Drawing for the job (mm, zero at the part's lowest x, y, z). Give positions to 0.01 mm unless a question says otherwise; leave off trailing zeros. Write each loop counter-clockwise with the first axis right and the second up, starting at its lowest first coordinate (ties: lowest second). Pieces come first, ordered by that corner, then holes. Notation, with made-up numbers: (46.5, 37.5) - (70.5, 37.5) arc R16 cw to (70.5, 59.5) - close; hole circle Ø9 at (6.25, -27.5). An arc over 180 degrees is marked (long way). Use CSV: the item, a comma, the result in double quotes.
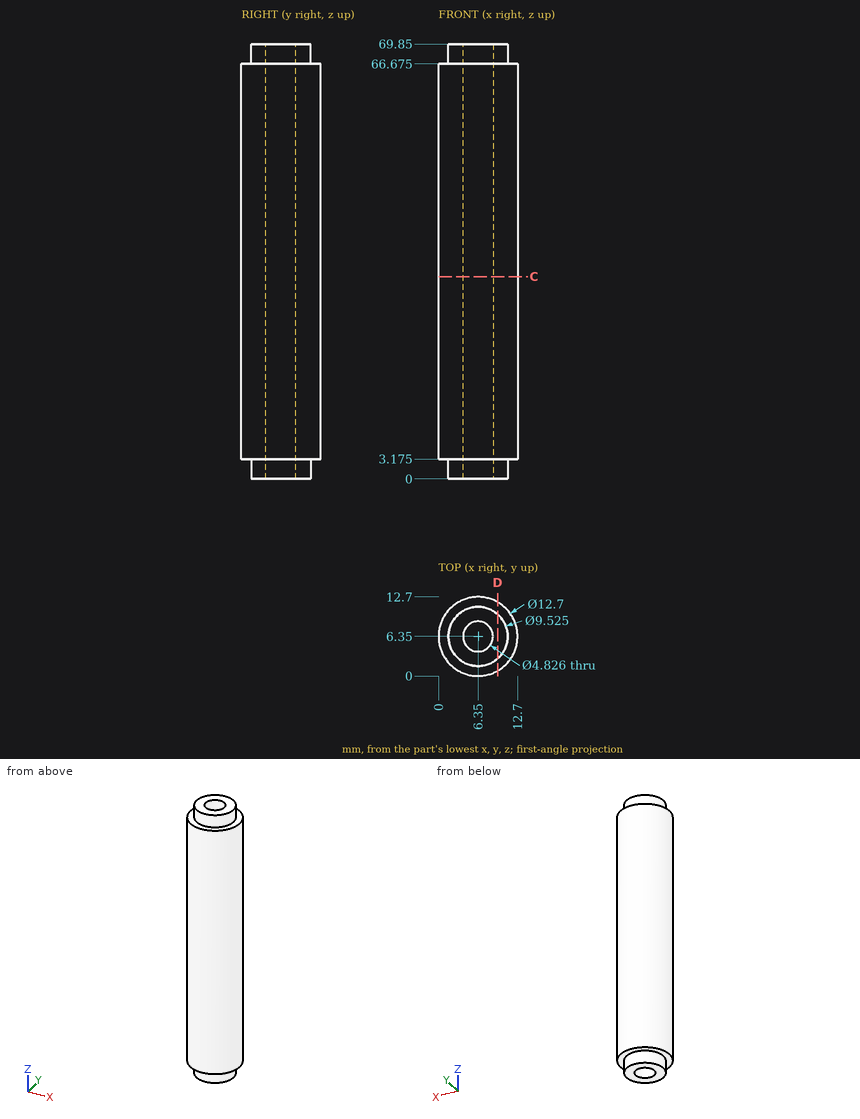
(1) Saw through at C-C, the plane z = 32.5. List the corners of the cut face in (x, y), then the cut area to 3 significant figures.
Checked values:
outline,"circle Ø12.7 at (6.35, 6.35); hole circle Ø4.83 at (6.35, 6.35)"
area,"108 mm^2"
(2) Saw through at D-D, the plane x = 9.5. List the corners of the cut face in (y, z) (3 decimals).
Checked values:
outline,"(0.836, 3.175) - (2.778, 3.175) - (2.778, 0) - (9.922, 0) - (9.922, 3.175) - (11.864, 3.175) - (11.864, 66.675) - (9.922, 66.675) - (9.922, 69.85) - (2.778, 69.85) - (2.778, 66.675) - (0.836, 66.675) - close"
(3) Wall check: probe 1 along Y at (x, z) = (6.35, 45.5); probe 2 along Z at (x, y) = (1.5, 7.5) (3 decimals); probe 3 along Y at (x, z) = (4.25, 27). Give the ranges that are in metal, low to high. Write a range as [from, to].
Checked values:
probe 1,"y = [0, 3.94], [8.76, 12.7]"
probe 2,"z = [3.175, 66.675]"
probe 3,"y = [0.36, 5.16], [7.54, 12.34]"
(4) Flat gauge pins, fed straight in: P1, Ø3, axis at x = 11, z = 18.5, coming from the -Y side; P2, Ø4, axis at x = 2, z = 17, coming from the +Y side; P3, Ø2, axis at x = 1.5, z = 56.5, coming from the -Y side. Where does each tip first touch, or does it go through?
Checked values:
P1,"stops at y = 0.84"
P2,"stops at y = 12.25"
P3,"stops at y = 1.3"
